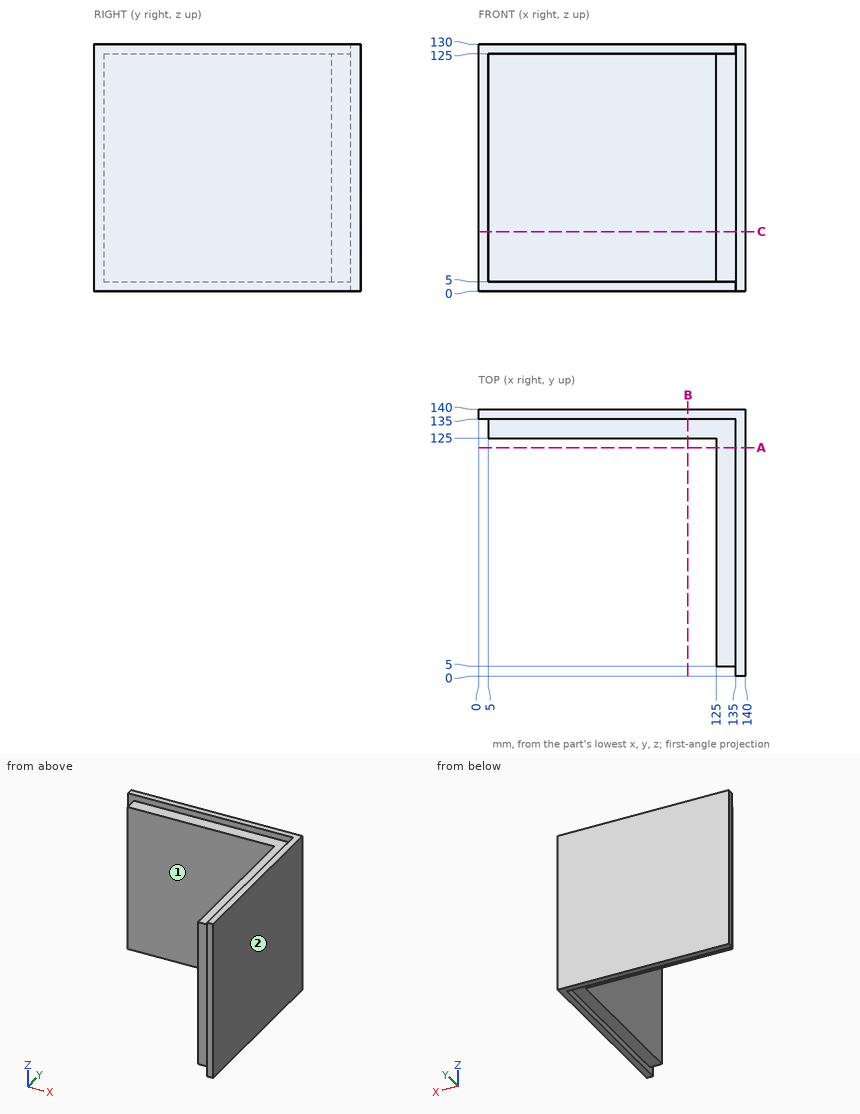
Geometry check sheet. Reference: drawing and pictorial views, mm from the part's lowest x, y, z. A direction names the side the tool comes from. Give positions to 0.01 mm unless a question says otherwise; leave off trailing zeros. Write each loop counter-clockwise with the first axis right and the second up, starting at its lowest first coordinate (ties: lowest second). Pieces come first, ordered by that corner, then holes.
Item 1: Cross-section at C-C (z = 31.5). Enter the section's corners in (x, y), and give its area (4 significant figures).
Item 2: Scan lines: L1, parallel to X at y = 69, z = 80; L2, parallel to Z at x = 27.5, y = 134. Record each from-to range of solid material in increasing order.
Item 3: Gauge pin test, flat ends, axial feed: pin 1 (10 mm diameter, centred on x = 43.5, z = 73, fed in from -Y); pin 2 (5 mm diameter, centred on y = 129.5, z = 55, fed in from -X); pin 3 (1.5 mm diameter, centred on y = 78, z = 57, fed in from -X). Record the tip position at first contact, or that the pin passes through.
Item 4: Access from +Z, -Z, +X, -X, +Y, -Y to the whole of each face (thin tool, end or side, straight path). Record for the marked faces 1 and 2.
Item 5: Cross-section at A-A (y = 120). Enter the section's corners in (x, z), and give its area (3 significant figures).
Report:
1. outline: (0, 135) - (5, 135) - (5, 125) - (125, 125) - (125, 5) - (135, 5) - (135, 0) - (140, 0) - (140, 140) - (0, 140) - close
1. area: 3,875 mm2
2. L1: x = 125 to 140
2. L2: z = 5 to 125
3. pin 1: stops at y = 125
3. pin 2: stops at x = 5
3. pin 3: stops at x = 125
4. face 1: +Z, -Z, -X, -Y
4. face 2: +Z, -Z, +X, +Y, -Y
5. outline: (125, 5) - (135, 5) - (135, 0) - (140, 0) - (140, 130) - (135, 130) - (135, 125) - (125, 125) - close
5. area: 1,850 mm2
